Geometry check sheet. Reference: the model listing, model coordinates, mm. Face numbers are marked on the shaded views. A direction names the side the tool comes from. Round coordinates to 2 decimals unless told otherwise and drop trailing zeros. Loops run counter-clockwise (first coordinate to the right, second up) from the corner with the lowest first, then second, coordinate; pieces in that order, holes last. Notation, with made-up numbers: M 74.25,33 L 118.25,33 A17 cw 118.25,65 Z; hole C -20,-11.5 d9. An arc over 180 degrees is marked long. Write item = value, one per line.
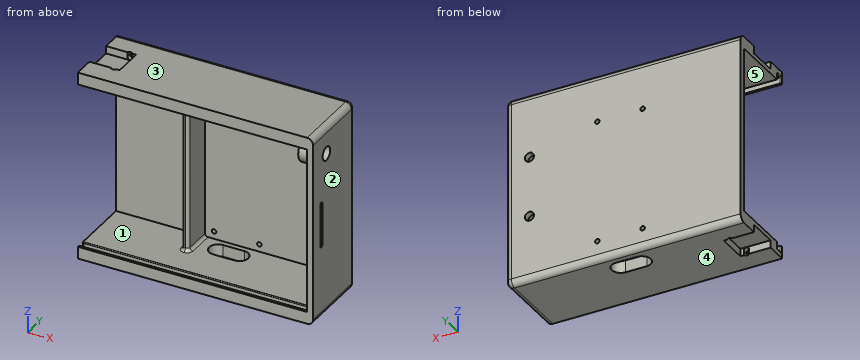
from build123d import *

# Parameters (mm, degrees)
SKETCH1_W               = 80
SKETCH1_H               = 63
BOSS_EXTRUDE2_DEPTH     = 25
SKETCH1_4_W             = 76
SKETCH1_4_H             = 55
CUT_EXTRUDE1_DEPTH      = 23
CUT_EXTRUDE2_DEPTH      = 20
SKETCH4_W               = 2
SKETCH4_H               = 55
BOSS_EXTRUDE3_DEPTH     = 10
FILLET1_R               = 2
SKETCH5_W               = 2
SKETCH5_H               = 63
CUT_EXTRUDE3_DEPTH      = 105.852277038
SKETCH6_W               = 2.2
SKETCH6_H               = 2.2
CUT_EXTRUDE4_DEPTH      = 76
SKETCH7_W               = 10
SKETCH7_H               = 10
CUT_EXTRUDE5_DEPTH      = 2.5
CUT_EXTRUDE6_DEPTH      = 11.5
CUT_EXTRUDE6_DEPTH_BACK = 1.5
SKETCH8_R               = 0.875
SKETCH9_W               = 10
SKETCH9_H               = 10
CUT_EXTRUDE7_DEPTH      = 2.5
CUT_EXTRUDE8_DEPTH      = 11.5
CUT_EXTRUDE8_DEPTH_BACK = 1.5
SKETCH10_R              = 0.875
CUT_EXTRUDE9_DEPTH      = 2
CUT_EXTRUDE10_DEPTH     = 2
SKETCH13_R              = 0.75
CUT_EXTRUDE11_DEPTH     = 105.393486469
FILLET2_R               = 0.3
CUT_EXTRUDE13_REACH     = 86.524
SKETCH15_W              = 5
SKETCH15_H              = 10
FILLET3_R               = 1
SKETCH16_R              = 4.25
BOSS_EXTRUDE4_DEPTH     = 5
CUT_EXTRUDE14_DEPTH     = 10
SKETCH21_R              = 1.5
CUT_EXTRUDE15_DEPTH     = 10


with BuildPart() as part:
    # Sketch1 → Boss-Extrude2 (new body)
    with BuildSketch(Plane(origin=(0, 0, 0), x_dir=(1, 0, 0), z_dir=(0, 1, 0))):
        with Locations((40, 31.5)):
            Rectangle(SKETCH1_W, SKETCH1_H)
    extrude(amount=BOSS_EXTRUDE2_DEPTH)

    # Sketch1<4> → Cut-Extrude1 (cut)
    with BuildSketch(Plane(origin=(0, 0, 0), x_dir=(1, 0, 0), z_dir=(0, 1, 0))):
        with Locations((40, 31.5)):
            Rectangle(SKETCH1_4_W, SKETCH1_4_H)
    extrude(amount=CUT_EXTRUDE1_DEPTH, mode=Mode.SUBTRACT)

    # Sketch3 → Cut-Extrude2 (cut)
    with BuildSketch(Plane(origin=(80, 0, 0), x_dir=(0, 0, -1), z_dir=(1, 0, 0))):
        with BuildLine():
            Line((38.5, 4.4), (24.5, 4.4))
            ThreePointArc((24.5, 4.4), (23.9, 5), (24.5, 5.6))
            Line((24.5, 5.6), (38.5, 5.6))
            ThreePointArc((38.5, 5.6), (39.1, 5), (38.5, 4.4))
        make_face()
    extrude(amount=-CUT_EXTRUDE2_DEPTH, mode=Mode.SUBTRACT)

    # Sketch4 → Boss-Extrude3 (add)
    with BuildSketch(Plane.XZ.offset(-23)):
        with Locations((30.5, -31.5)):
            Rectangle(SKETCH4_W, SKETCH4_H)
    extrude(amount=BOSS_EXTRUDE3_DEPTH)

    # Fillet1
    fillet1_edges = [part.edges().sort_by_distance(p)[0] for p in [
        (80, 25, -31.5),
        (40, 25, 0),
        (0, 25, -31.5),
        (0, 12.5, 0),
        (80, 12.5, 0),
        (80, 12.5, -63),
        (0, 12.5, -63),
        (40, 25, -63),
    ]]
    fillet(fillet1_edges, radius=FILLET1_R)

    # Sketch5 → Cut-Extrude3 (cut, through all)
    with BuildSketch(Plane(origin=(0, 0, 0), x_dir=(-1, 0, 0), z_dir=(0, -1, 0))):
        with Locations((-1, 31.5)):
            Rectangle(SKETCH5_W, SKETCH5_H)
    extrude(amount=-CUT_EXTRUDE3_DEPTH, mode=Mode.SUBTRACT)

    # Sketch6 → Cut-Extrude4 (cut)
    with BuildSketch(Plane.ZY.offset(-2)):
        with Locations((-2.9, 1.85)):
            Rectangle(SKETCH6_W, SKETCH6_H)
        with Locations((-60.1, 1.85)):
            Rectangle(SKETCH6_W, SKETCH6_H)
    extrude(amount=-CUT_EXTRUDE4_DEPTH, mode=Mode.SUBTRACT)

    # Sketch7 → Cut-Extrude5 (cut)
    with BuildSketch(Plane(origin=(0, 0, -63), x_dir=(-1, 0, 0), z_dir=(0, 0, -1))):
        with Locations((-7, 12)):
            Rectangle(SKETCH7_W, SKETCH7_H)
    extrude(amount=-CUT_EXTRUDE5_DEPTH, mode=Mode.SUBTRACT)

    # Sketch8 → Cut-Extrude6 (cut, two sides: drawn at the far end of the back side and taken through both)
    with BuildSketch(Plane(origin=(0, 7, 0), x_dir=(1, 0, 0), z_dir=(0, 1, 0)).offset(-CUT_EXTRUDE6_DEPTH_BACK)):
        with Locations(Location((10, 61.5, 0), (0, 0, 270))):
            Circle(SKETCH8_R)
    extrude(amount=CUT_EXTRUDE6_DEPTH + CUT_EXTRUDE6_DEPTH_BACK, mode=Mode.SUBTRACT)

    # Sketch9 → Cut-Extrude7 (cut)
    with BuildSketch(Plane.XY):
        with Locations((7, 12)):
            Rectangle(SKETCH9_W, SKETCH9_H)
    extrude(amount=-CUT_EXTRUDE7_DEPTH, mode=Mode.SUBTRACT)

    # Sketch10 → Cut-Extrude8 (cut, two sides: drawn at the far end of the back side and taken through both)
    with BuildSketch(Plane(origin=(0, 7, 0), x_dir=(1, 0, 0), z_dir=(0, 1, 0)).offset(-CUT_EXTRUDE8_DEPTH_BACK)):
        with Locations((10, 1.5)):
            Circle(SKETCH10_R)
    extrude(amount=CUT_EXTRUDE8_DEPTH + CUT_EXTRUDE8_DEPTH_BACK, mode=Mode.SUBTRACT)

    # Sketch11 → Cut-Extrude9 (cut)
    with BuildSketch(Plane(origin=(0, 0, -63), x_dir=(-1, 0, 0), z_dir=(0, 0, -1))):
        with BuildLine():
            Line((-9.122986176, 7), (-10.8, 7))
            add(Edge.make_bspline(
                [(-10.8, 7), (-10.004539285, 5.994886644), (-9.122986176, 7)],
                knots=[0, 0, 0, 1, 1, 1], degree=2))
        make_face()
        with BuildLine():
            Line((-9.122986176, 17), (-10.8, 17))
            add(Edge.make_bspline(
                [(-10.8, 17), (-10.004539285, 18.005113356), (-9.122986176, 17)],
                knots=[0, 0, 0, 1, 1, 1], degree=2))
        make_face()
    extrude(amount=-CUT_EXTRUDE9_DEPTH, mode=Mode.SUBTRACT)

    # Sketch12 → Cut-Extrude10 (cut)
    with BuildSketch(Plane.XY):
        with BuildLine():
            Line((10.8, 7), (9.120131213, 7))
            add(Edge.make_bspline(
                [(10.8, 7), (10.003016043, 5.994891859), (9.120131213, 7)],
                knots=[0, 0, 0, 1, 1, 1], degree=2))
        make_face()
        with BuildLine():
            Line((10.8, 17), (9.120131213, 17))
            add(Edge.make_bspline(
                [(10.8, 17), (10.003016043, 18.005108141), (9.120131213, 17)],
                knots=[0, 0, 0, 1, 1, 1], degree=2))
        make_face()
    extrude(amount=-CUT_EXTRUDE10_DEPTH, mode=Mode.SUBTRACT)

    # Sketch13 → Cut-Extrude11 (cut, through all)
    with BuildSketch(Plane(origin=(0, 23, 0), x_dir=(-1, 0, 0), z_dir=(0, -1, 0))):
        with Locations(Location((-34.5, 56.5, 0), (0, 0, 90))):
            Circle(SKETCH13_R)
        with Locations(Location((-49.5, 56.5, 0), (0, 0, 90))):
            Circle(SKETCH13_R)
        with Locations(Location((-34.5, 16, 0), (0, 0, 90))):
            Circle(SKETCH13_R)
        with Locations(Location((-49.5, 16, 0), (0, 0, 90))):
            Circle(SKETCH13_R)
    extrude(amount=-CUT_EXTRUDE11_DEPTH, mode=Mode.SUBTRACT)

    # Fillet2
    fillet2_edges = [part.edges().sort_by_distance(p)[0] for p in [
        (40, 2.95, -59),
        (2, 0.75, -60.1),
        (2, 1.85, -61.2),
        (40, 0.75, -61.2),
        (40, 2.95, -61.2),
        (2, 2.95, -60.1),
        (2, 2.95, -2.9),
        (40, 2.95, -4),
        (40, 2.95, -1.8),
        (40, 0.75, -1.8),
        (2, 0.75, -2.9),
        (2, 1.85, -1.8),
    ]]
    fillet(fillet2_edges, radius=FILLET2_R)

    # Sketch15 → Cut-Extrude13 (cut, up to next)
    with BuildSketch(Plane.ZY.offset(-29.5), mode=Mode.PRIVATE) as cut_extrude13_sk1:
        with Locations((-6.5, 18)):
            Rectangle(SKETCH15_W, SKETCH15_H)
    cut_extrude13_tool1 = extrude(cut_extrude13_sk1.sketch, amount=-CUT_EXTRUDE13_REACH, mode=Mode.PRIVATE) & part.part
    add(cut_extrude13_tool1.solids().sort_by_distance((29.5, 18, -6.5))[0], mode=Mode.SUBTRACT)

    # Fillet3
    fillet3_edges = [part.edges().sort_by_distance(p)[0] for p in [
        (29.5, 13, -34),
        (30.5, 13, -9),
        (29.5, 18, -59),
        (31.5, 18, -59),
        (30.5, 13, -59),
        (31.5, 13, -34),
    ]]
    fillet(fillet3_edges, radius=FILLET3_R - 0.0001)  # a hair under: the kernel refuses the full size

    # Sketch16 → Boss-Extrude4 (add)
    with BuildSketch(Plane.ZY.offset(-78)):
        with Locations((-9, 8)):
            Circle(SKETCH16_R)
    extrude(amount=BOSS_EXTRUDE4_DEPTH)

    # Cut-Loft1: read off the stored shape, not the designer's step
    # Cut-Loft1: loft between two sections, ruled curve by curve
    cut_loft1_from = [
        Edge.make_bspline([(73, 5.618142213, -10.374501175), (73, 8.367144563, -15.13821675), (73, 13.130860138, -12.3892144), (73, 10.381857787, -7.625498825), (73, 7.632855437, -2.86178325), (73, 2.869139862, -5.6107856), (73, 5.618142213, -10.374501175)], [0, 0, 0, 0, 0.5, 0.5, 0.5, 1, 1, 1, 1], 3, [1, 0.333333333, 0.333333333, 1, 0.333333333, 0.333333333, 1]),
    ]
    cut_loft1_to = [
        Edge.make_bspline([(80, 6.404019358, -10.585984171), (80, 9.575987701, -13.777945454), (80, 12.767948984, -10.605977112), (80, 9.595980642, -7.414015829), (80, 6.424012299, -4.222054546), (80, 3.232051016, -7.394022888), (80, 6.404019358, -10.585984171)], [0, 0, 0, 0, 0.5, 0.5, 0.5, 1, 1, 1, 1], 3, [1, 0.333333333, 0.333333333, 1, 0.333333333, 0.333333333, 1]),
    ]
    cut_loft1 = Solid(Shell([*[Face.make_surface_from_curves(cut_loft1_from[k], cut_loft1_to[k]) for k in range(1)], Face(Wire(cut_loft1_from)), Face(Wire(cut_loft1_to))]))
    add(cut_loft1, mode=Mode.SUBTRACT)

    # Sketch20 → Cut-Extrude14 (cut)
    with BuildSketch(Plane(origin=(0, 0, -63), x_dir=(-1, 0, 0), z_dir=(0, 0, -1))):
        with BuildLine():
            Line((-38.5, 15.2), (-45.5, 15.2))
            ThreePointArc((-45.5, 15.2), (-48.5, 18.2), (-45.5, 21.2))
            Line((-45.5, 21.2), (-38.5, 21.2))
            ThreePointArc((-38.5, 21.2), (-35.5, 18.2), (-38.5, 15.2))
        make_face()
    extrude(amount=-CUT_EXTRUDE14_DEPTH, mode=Mode.SUBTRACT)

    # Sketch21 → Cut-Extrude15 (cut)
    with BuildSketch(Plane.XZ.offset(-23)):
        with Locations(Location((72, -41.5, 0), (0, 0, 270))):
            Circle(SKETCH21_R)
        with Locations(Location((72, -21.5, 0), (0, 0, 270))):
            Circle(SKETCH21_R)
    extrude(amount=-CUT_EXTRUDE15_DEPTH, mode=Mode.SUBTRACT)


solid = part.part
(1) Depth check by flat-ended pin: pin 1 Ø16.5 at (x, z) = (55, -26.5) entering from -Y; pin 2 Ø2.5 at (y, z) = (8.5, -10.5) entering from -X. Enter the tip coordinate at first touch or a pass-through.
Result set:
pin_1 = 23
pin_2 = 73
(2) Sectioned sample at C-C on x = 72. State how many separate pieces and enclosed holes the cut face has, then the cut area to 3 significant figures.
Result set:
separate_pieces = 3
enclosed_holes = 0
area = 287 mm2
(3) Release check for a two-part mould opening along X. For the marked faces 1, 2 and 3 record: released by +X, released by -X, zero draft, split by the parting line, or undercut.
Result set:
face_1 = undercut
face_2 = released by +X
face_3 = zero draft
(4) Material ranges on line 1 along Z through (x, y) = (10, 17.95) (3 decimals); line 2 along Z through (x, y) = (74, 16.75); line 3 along Z through (x, y) = (72, 24.45), recorded low to high. Write a range as from..to.
Result set:
line_1 = -63..-62.375, -60.625..-59, -4..-2.375, -0.625..0
line_2 = -63..-59, -4..0
line_3 = -62.38..-43, -40..-23, -20..-0.62
(5) Tool access check on the marked faces 4 and 5. Record the directions out of +Z, -Z, +X, -X, +Y, -Y that give a thin tool (end or side, any length) a straight path to the whole face; none if there is none.
Result set:
face_4 = -Z, +X, -X, +Y, -Y
face_5 = -X, -Y
(6) Sectioned sample at A-A on x = 24. Record the cut outline in (y, z).
Result set:
outline = M 0,-63 L 23,-63 A2 ccw 25,-61 L 25,-2 A2 ccw 23,0 L 0,0 L 0,-4 L 0.75,-4 L 0.75,-2.1 A0.3 cw 1.05,-1.8 L 2.65,-1.8 A0.3 cw 2.95,-2.1 L 2.95,-3.7 A0.3 ccw 3.25,-4 L 23,-4 L 23,-59 L 3.25,-59 A0.3 ccw 2.95,-59.3 L 2.95,-60.9 A0.3 cw 2.65,-61.2 L 1.05,-61.2 A0.3 cw 0.75,-60.9 L 0.75,-59 L 0,-59 Z
